Autodesk Fusion 360 part; units mm, degrees
sketch "Esquisse1" plane through (0, 0, 0) normal (0, 1, 0) x (1, 0, 0)
  line L0 (30, -20) -> (20, -20)
  line L1 (20, -20) -> (20, -10)
  line L2 (20, -10) -> (30, -10)
  line L3 (30, -10) -> (30, -20)
  circle A0 centre (25, -15) radius 1
  dimension "d1" = 10
  dimension "d2" = 10
  dimension "d22" = 2
extrude "Extrusion3" add sketch "Esquisse1" along normal blind 4
sketch "Esquisse3" plane through (0, 4, 0) normal (0, 1, 0) x (-1, 0, 0)
  circle A0 centre (-25, 15) radius 1
  line L0 (-30, 10) -> (-20, 10)
  line L1 (-20, 10) -> (-20, 20)
  line L2 (-20, 20) -> (-30, 20)
  line L3 (-30, 20) -> (-30, 10)
  line L4 (-30, 20) -> (-30, 17)
  line L5 (-30, 17) -> (-27.5, 17)
  line L6 (-27.5, 17) -> (-27.5, 15)
  line L7 (-27.5, 15) -> (-27, 15)
  line L8 (-25, 16.75) -> (-25, 17.5)
  line L9 (-25, 17.5) -> (-27, 17.5)
  line L10 (-27, 17.5) -> (-27, 20)
  line L11 (-27, 20) -> (-30, 20)
  line L12 (-30, 17) -> (-30, 20)
  line L13 (-26.75, 15) -> (-27.625, 15)
  line L14 (-25, 17.5) -> (-25, 17)
  line L15 (-25, 16.75) -> (-26.75, 16.75)
  line L16 (-26.75, 16.75) -> (-26.75, 15)
  line L17 (-27.5, 13) -> (-30, 13)
  line L18 (-30, 13) -> (-30, 10)
  line L19 (-30, 10) -> (-27, 10)
  line L20 (-27, 12.5) -> (-25, 12.5)
  line L21 (-25, 12.5) -> (-25, 13)
  line L22 (-27, 10) -> (-27, 12.5)
  line L23 (-25, 13.25) -> (-25, 12.375)
  line L24 (-26.75, 13.25) -> (-25, 13.25)
  line L25 (-26.75, 15) -> (-26.75, 13.25)
  line L26 (-26.75, 15) -> (-27.5, 15)
  line L27 (-27.5, 15) -> (-27.5, 13)
  line L28 (-23, 12.5) -> (-23, 10)
  line L29 (-23, 10) -> (-20, 10)
  line L30 (-20, 10) -> (-20, 13)
  line L31 (-22.5, 13) -> (-22.5, 15)
  line L32 (-22.5, 15) -> (-23, 15)
  line L33 (-20, 13) -> (-22.5, 13)
  line L34 (-23.25, 15) -> (-22.375, 15)
  line L35 (-23.25, 13.25) -> (-23.25, 15)
  line L36 (-25, 13.25) -> (-23.25, 13.25)
  line L37 (-25, 13.25) -> (-25, 12.5)
  line L38 (-25, 12.5) -> (-23, 12.5)
  line L39 (-22.5, 17) -> (-20, 17)
  line L40 (-20, 17) -> (-20, 20)
  line L41 (-20, 20) -> (-23, 20)
  line L42 (-23, 17.5) -> (-25, 17.5)
  line L43 (-25, 17.5) -> (-25, 17)
  line L44 (-23, 20) -> (-23, 17.5)
  line L45 (-25, 16.75) -> (-25, 17.625)
  line L46 (-23.25, 16.75) -> (-25, 16.75)
  line L47 (-23.25, 15) -> (-23.25, 16.75)
  line L48 (-23.25, 15) -> (-22.5, 15)
  line L49 (-22.5, 15) -> (-22.5, 17)
  dimension "d19" = 2.5
  dimension "d20" = 2
  dimension "d21" = 2.5
  dimension "d25" = 360
  dimension "d27" = 0.75
  dimension "d28" = 0.75
  dimension "d36" = 4
  dimension "d37" = 3
  dimension "d38" = 3
extrude "Extrusion6" add sketch "Esquisse3" along normal blind 46 contours L0 L3 L7 L13 L17 L18 L19 L20 L21 L22 L23 L24 L25 L26 L27 L37 | L0 L1 L21 L23 L28 L29 L30 L31 L32 L33 L34 L35 L36 L37 L38 L48 | L2 L3 L4 L5 L6 L7 L8 L9 L10 L11 L12 L13 L14 L15 L16 L26 L43 L45 | L1 L2 L8 L14 L32 L34 L39 L40 L41 L42 L43 L44 L45 L46 L47 L48 L49
fillet "Congé2" radius 1 4 edges at (23.25, 27, 13.25) (26.75, 27, 13.25) (26.75, 27, 16.75) (23.25, 27, 16.75)
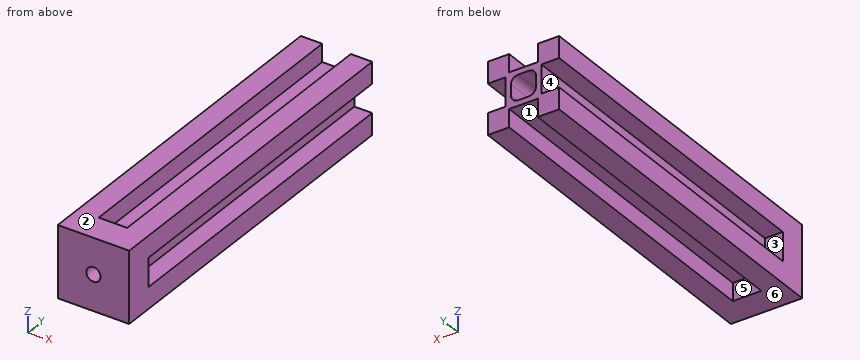
Geometry: final body of the model. Coordinates: model frame, mm. Face numbers are marked on the shaded views. A direction names the side the tool comes from. Give positions to 0.01 mm unless a question says otherwise; leave off trailing zeros. Write each loop counter-clockwise with the first axis right and the second up, starting at its lowest first coordinate (ties: lowest second). Pieces come first, ordered by that corner, then holes. Notation, with made-up numbers: (-33.75, 43) -> (11.25, 43) arc R18 cw to (11.25, 55) -> close; hole circle Ø1 at (28, 14.5). An arc over 180 degrees is marked (long way). Answer in a Markdown table with one row per item.
(1) Section query B-B on z = 15. Return loops of the section in (x, y).
Answers below:
| item | result |
|---|---|
| outline | (20, 0) -> (24, 0) -> (24, 4) -> (23.25, 4) -> (23.25, 50) -> (22.5, 50) -> (22.5, 4) -> (20, 4) -> close; (26, 0) -> (30, 0) -> (30, 4) -> (27.5, 4) -> (27.5, 50) -> (26.75, 50) -> (26.75, 4) -> (26, 4) -> close |
(2) Section query A-A on y = 11. Return loops of the section in (x, z), then the cut area to 3 significant figures.
Answers below:
| item | result |
|---|---|
| outline | (20, 10) -> (23, 10) -> (23, 12.5) -> (27, 12.5) -> (27, 10) -> (30, 10) -> (30, 13) -> (27.5, 13) -> (27.5, 17) -> (30, 17) -> (30, 20) -> (27, 20) -> (27, 17.5) -> (23, 17.5) -> (23, 20) -> (20, 20) -> (20, 17) -> (22.5, 17) -> (22.5, 13) -> (20, 13) -> close; hole (23.25, 14.25) arc R1 ccw to (24.25, 13.25) -> (25.75, 13.25) arc R1 ccw to (26.75, 14.25) -> (26.75, 15.75) arc R1 ccw to (25.75, 16.75) -> (24.25, 16.75) arc R1 ccw to (23.25, 15.75) -> close |
| area | 48.6 mm^2 |
(3) Draft query along Z for the marked faces 1, 2, 3 and 4. Return one class per face: +Z half, -Z half, draft (parallel to the pull), parting line (faces both ways), or undercut.
Answers below:
| item | result |
|---|---|
| face 1 | -Z half |
| face 2 | +Z half |
| face 3 | undercut |
| face 4 | undercut |
(4) Set-up query: the marked faces 5 and 6. Return all of +Z, -Z, +X, -X, +Y, -Y with unobstructed straight access to the full face (end or side cutting, diameter ignored); none if empty.
Answers below:
| item | result |
|---|---|
| face 5 | -Z, +Y |
| face 6 | -Z, +X, -X, +Y, -Y |
(5) Ray query, line 1 along Z through (x, y) = (20.75, 20); line 2 along X through (y, z) = (2.3, 15); line 3 along Z through (x, y) = (25, 0.9). Return the intervals inside material, ascending. Write a range as [from, to].
Answers below:
| item | result |
|---|---|
| line 1 | [10, 13], [17, 20] |
| line 2 | [20, 24], [26, 30] |
| line 3 | [10, 14], [16, 20] |
(6) Pin query (flat end, axial travel): pin 1 (2 mm diameter, centred on y = 33.5, z = 14.5, fed in from -X); pin 2 (1.5 mm diameter, centred on x = 25, y = 36.5, fed in from -Z); pin 3 (1.5 mm diameter, centred on y = 22.5, z = 14, fed in from +X). Return the tip coordinate at first contact, or that it passes through.
Answers below:
| item | result |
|---|---|
| pin 1 | x = 22.5 |
| pin 2 | z = 12.5 |
| pin 3 | x = 27.5 |
(7) Section query C-C on x = 25. Return loops of the section in (y, z).
Answers below:
| item | result |
|---|---|
| outline | (0, 10) -> (4, 10) -> (4, 12.5) -> (50, 12.5) -> (50, 13.25) -> (4, 13.25) -> (4, 14) -> (0, 14) -> close; (0, 16) -> (4, 16) -> (4, 16.75) -> (50, 16.75) -> (50, 17.5) -> (4, 17.5) -> (4, 20) -> (0, 20) -> close |
(8) Section query D-D on x = 21.5. Return loops of the section in (y, z), then the cut area to 3 significant figures.
Answers below:
| item | result |
|---|---|
| outline | (0, 10) -> (50, 10) -> (50, 13) -> (4, 13) -> (4, 17) -> (50, 17) -> (50, 20) -> (0, 20) -> close |
| area | 316 mm^2 |
